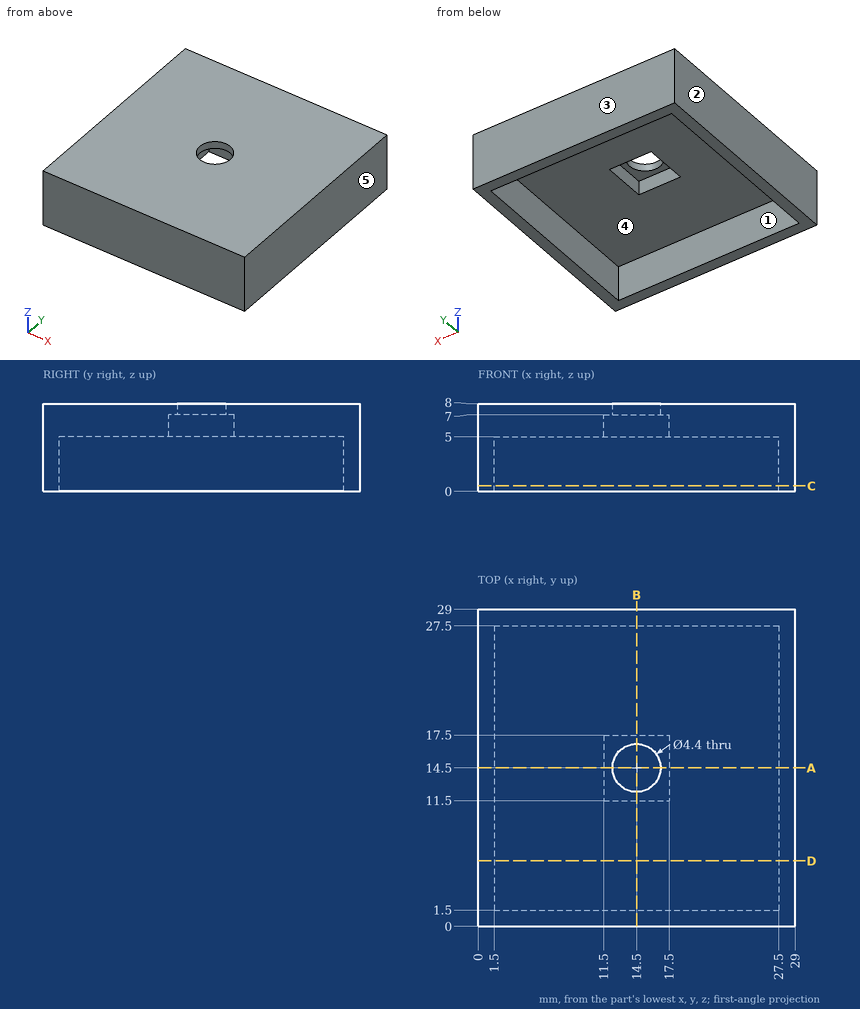
Answer from the drawing. Dimensions are ordinates in mm from the lowest x, y and z of the part. A direction names the side the tool comes from. Coordinates: 2 decimals unless noted, no trailing zeros. Loops run counter-clockwise (first coordinate to the right, second up) from the corner with the lowest first, then second, coordinate; pieces in that order, holes last. Notation, with made-up numbers: (-2, 64) - (22, 64) arc R16 ccw to (22, 95) - close; hole circle Ø2 at (-14, 19.5). An arc over 180 degrees is marked (long way). Use a Markdown table: item, result.
Item 1: The mould has two halves that part along X. Classify the marked faces 3, 4 and 5: +X half, -X half, draft (parallel to the pull), parting line (faces both ways), or undercut.
Evaluation:
| item | result |
|---|---|
| face 3 | draft |
| face 4 | undercut |
| face 5 | +X half |
Item 2: Consider probe 1 along X at (y, z) = (14.5, 7.55); probe 2 along Y at (x, z) = (9.75, 1.75). Determine where each line is inside the solid, lowest interval first. Write a range as from..to.
Evaluation:
| item | result |
|---|---|
| probe 1 | x = 0..12.3, 16.7..29 |
| probe 2 | y = 0..1.5, 27.5..29 |
Item 3: Find section D-D, the plane y = 6. Determine the outline of the cut face in (x, z).
Evaluation:
| item | result |
|---|---|
| outline | (0, 0) - (1.5, 0) - (1.5, 5) - (27.5, 5) - (27.5, 0) - (29, 0) - (29, 8) - (0, 8) - close |
Item 4: Given pin 1 Ø6 at (x, y) = (10, 17) entering from -Z, flat-ended and moving along its own axis, determine where the tip first touches the part or whether it passes through.
Evaluation:
| item | result |
|---|---|
| pin 1 | stops at z = 5 |
Item 5: Find section A-A, the plane y = 14.5. Determine the outline of the cut face in (x, z).
Evaluation:
| item | result |
|---|---|
| outline | (0, 0) - (1.5, 0) - (1.5, 5) - (11.5, 5) - (11.5, 7) - (12.3, 7) - (12.3, 8) - (0, 8) - close; (16.7, 7) - (17.5, 7) - (17.5, 5) - (27.5, 5) - (27.5, 0) - (29, 0) - (29, 8) - (16.7, 8) - close |
Item 6: Find section C-C, the plane z = 0.5. Determine the outline of the cut face in (x, y), and give its area (3 significant figures).
Evaluation:
| item | result |
|---|---|
| outline | (0, 0) - (29, 0) - (29, 29) - (0, 29) - close; hole (1.5, 1.5) - (27.5, 1.5) - (27.5, 27.5) - (1.5, 27.5) - close |
| area | 165 mm2 |
Item 7: For the marked faces 1 and 2, determine the directions among +Z, -Z, +X, -X, +Y, -Y from which every point of the face is accessible in a straight line to the end or side of a thin tool.
Evaluation:
| item | result |
|---|---|
| face 1 | -Z |
| face 2 | +Z, -Z, -X, +Y, -Y |
